For this review, use the dimensioned drawing (mm, ordinates from the lowest corner) and the shaded views. Coordinates: 2 decimals unless noted, no trailing zeros. Write each loop counter-clockwise with the first axis right and the second up, starting at its lowest first coordinate (ties: lowest second). Pieces come first, ordered by that corner, then holes. Notation, with made-up numbers: (-40, -2.5) - (4, -2.5) arc R21 ccw to (4, 2.5) - close; hole circle Ø8 at (33.25, 3). An arc over 180 degrees is marked (long way). Answer as a JSON object with one key per item and string values.
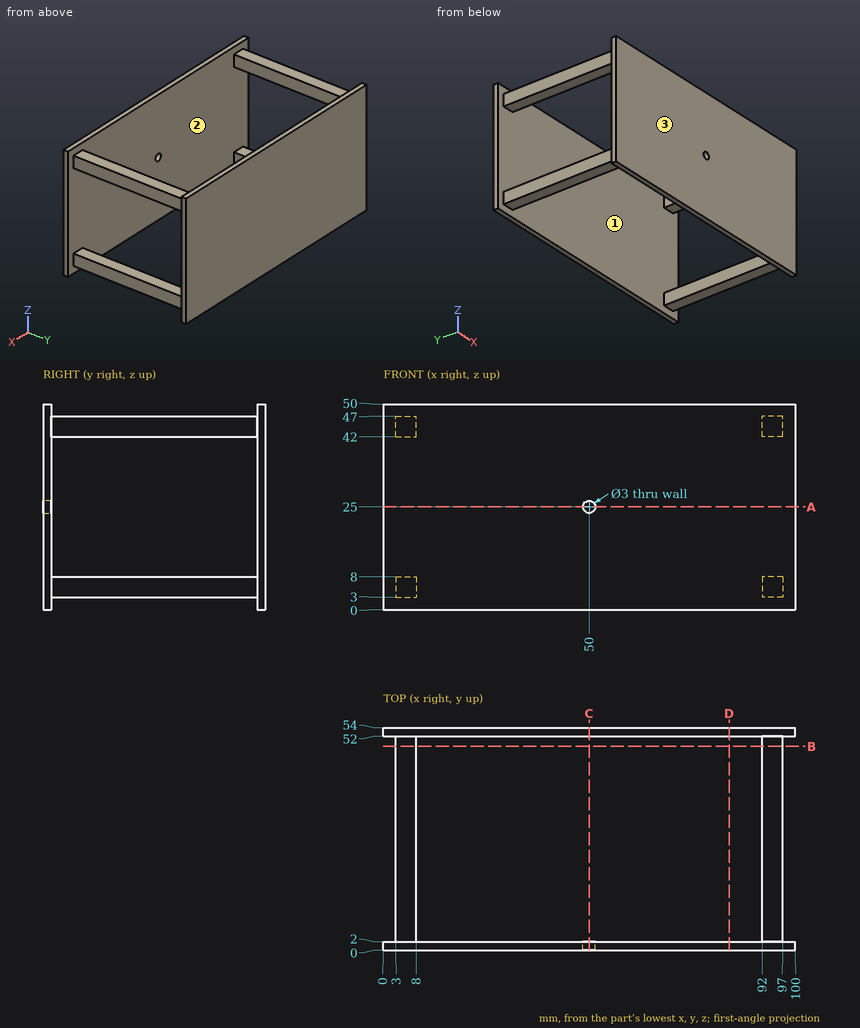
(1) For pin 1 (2.5 mm diameter, centred on y = 15, z = 5.5, fed in from -X); pin 2 (4 mm diameter, centred on y = 25, z = 6.5, fed in from +X); pin 3 (4 mm diameter, centred on x = 5.5, y = 19.5, fed in from -Z), all flat-tipped, find the tip position at first contact; note any pin that passes through.
Solved:
{"pin 1": "stops at x = 3", "pin 2": "stops at x = 97", "pin 3": "stops at z = 3"}
(2) Take a section at B-B, the plane y = 49.5. Write out the cut boundary in (x, z), and give its area (3 significant figures).
Solved:
{"outline": "(3, 3) - (8, 3) - (8, 8) - (3, 8) - close; (3, 42) - (8, 42) - (8, 47) - (3, 47) - close; (92, 3) - (97, 3) - (97, 8) - (92, 8) - close; (92, 42) - (97, 42) - (97, 47) - (92, 47) - close", "area": "100 mm^2"}
(3) To check wall thickness, follow line 1 (Z direction, x = 6, y = 5); line 2 (X direction, y = 1.1, z = 25); line 3 (Y direction, x = 83, z = 47.5). State the ranges of each line that lie inside material, in increasing order. Write a range as from..to.
Solved:
{"line 1": "z = 3..8, 42..47", "line 2": "x = 0..48.5, 51.5..100", "line 3": "y = 0..2, 52..54"}
(4) The part is to be moulded in two halves that separate along X. For the marked faces 1, 2 and 3, say which applies: pulls with the +X half, pulls with the -X half, needs draft (parallel to the pull), parting line crosses it, or undercut.
Solved:
{"face 1": "undercut", "face 2": "undercut", "face 3": "needs draft"}
(5) Take a section at A-A, the plane z = 25. Write out the cut boundary in (x, y), and give its area (3 significant figures).
Solved:
{"outline": "(0, 0) - (48.5, 0) - (48.5, 2) - (0, 2) - close; (0, 52) - (100, 52) - (100, 54) - (0, 54) - close; (51.5, 0) - (100, 0) - (100, 2) - (51.5, 2) - close", "area": "394 mm^2"}
(6) Take a section at C-C, the plane x = 50. Write out the cut boundary in (y, z), and give its area (3 significant figures).
Solved:
{"outline": "(0, 0) - (2, 0) - (2, 23.5) - (0, 23.5) - close; (0, 26.5) - (2, 26.5) - (2, 50) - (0, 50) - close; (52, 0) - (54, 0) - (54, 50) - (52, 50) - close", "area": "194 mm^2"}
(7) Take a section at D-D, the plane x = 84. Write out the cut boundary in (y, z).
Solved:
{"outline": "(0, 0) - (2, 0) - (2, 50) - (0, 50) - close; (52, 0) - (54, 0) - (54, 50) - (52, 50) - close"}
